Geometry: final body of the model. Coordinates: model frame, mm. Face numbers are marked on the shaded views. A direction names the side the tool comes from. Give positions to 0.01 mm unless a question says otherwise; leave off trailing zeros. Write each loop counter-clockwise with the first axis right and the second up, starting at its lowest first coordinate (ties: lowest second). Pieces come first, ordered by that corner, then holes.
Q1. Section B-B (y = 12.7). Return the cut outline in (x, z) (1 decimal).
Q2. Line query: line 1 (Y direction, x = 24.6, z = -5.92); line 2 (X direction, y = 0.75, z = 0) (3 decimals); line 3 (Y direction, x = 17.5, z = 7.25) (3 decimals). Output: solid intervals per line, ascending.
Q3. Reachability of the marked faces 1 and 2 from +Z, -Z, +X, -X, +Y, -Y: full face, straight path, thin tool, end or side. Return the list, or none.
Q4. Section C-C (x = 15). Return the cut outline in (y, z) (3 decimals), plus the area to 3 significant figures.
Q5. Section A-A (z = 0). State how many separate pieces and enclosed holes the cut face has, plus the area to 3 significant figures.
Q6. Pin query (flat end, axial travel): pin 1 Ø4 at (y, z) = (31.75, -5.92) entering from +X; pin 2 Ø4 at (x, z) = (15.58, 7.36) entering from +Y (3 decimals); pin 3 Ø2.5 at (x, z) = (15.58, -7.36) entering from -Y; pin 4 Ø12 at (y, z) = (15, 6.5) entering from -X (3 decimals). Return the tip coordinate at first contact, or that it passes through.
from build123d import *

# Parameters (mm, degrees)
BOSS_EXTRUDE1_DEPTH = 11
FILLET1_R           = 1.5875
SKETCH3_W           = 24.423912887
SKETCH3_H           = 26.552361768
CUT_EXTRUDE1_DEPTH  = 61.908127536
SKETCH4_R           = 1.5
SKETCH4_R_2         = 6.5
SKETCH4_W           = 25.825
SKETCH4_H           = 22
CUT_EXTRUDE2_DEPTH  = 53.363751775
SKETCH5_R           = 1.5875
CUT_EXTRUDE3_DEPTH  = 53.158921816


with BuildPart() as part:
    # Sketch2 → Boss-Extrude1 (new, symmetric)
    with BuildSketch(Plane.XY):
        Polygon((-25.4, 0), (25.4, 0), (25.4, 50.8), (22.225, 50.8), (22.225, 3.175), (-25.4, 3.175), align=None)
    extrude(amount=BOSS_EXTRUDE1_DEPTH, both=True)

    # Fillet1
    fillet1_edges = [part.edges().sort_by_distance(p)[0] for p in [
        (22.225, 3.175, 0),
    ]]
    fillet(fillet1_edges, radius=FILLET1_R)

    # Sketch3 → Cut-Extrude1 (cut, through all)
    with BuildSketch(Plane.XY.offset(11)):
        with Locations((18.271034128, 57.726180884)):
            Rectangle(SKETCH3_W, SKETCH3_H)
    extrude(amount=-CUT_EXTRUDE1_DEPTH, mode=Mode.SUBTRACT)

    # Sketch4 → Cut-Extrude2 (cut, through all)
    with BuildSketch(Plane.XZ):
        with Locations(Location((15.575, -7.361215932, 0), (0, 0, 270))):
            Circle(SKETCH4_R)
        with Locations(Location((11.325, 0, 0), (0, 0, 270))):
            Circle(SKETCH4_R_2)
        with Locations(Location((15.575, 7.361215932, 0), (0, 0, 270))):
            Circle(SKETCH4_R)
        with Locations((-12.4875, 0)):
            Rectangle(SKETCH4_W, SKETCH4_H)
        with Locations(Location((2.825, 0, 0), (0, 0, 270))):
            Circle(SKETCH4_R)
    extrude(amount=-CUT_EXTRUDE2_DEPTH, mode=Mode.SUBTRACT)

    # Sketch5 → Cut-Extrude3 (cut, through all)
    with BuildSketch(Plane(origin=(25.4, 0, 0), x_dir=(0, 0, -1), z_dir=(1, 0, 0))):
        with Locations((5.92, 31.75)):
            Circle(SKETCH5_R)
        with Locations((5.92, 12.7)):
            Circle(SKETCH5_R)
    extrude(amount=-CUT_EXTRUDE3_DEPTH, mode=Mode.SUBTRACT)


solid = part.part
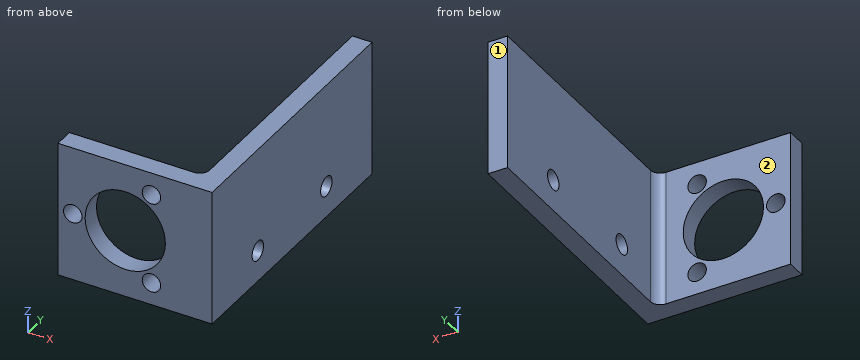
Computed:
1. outline: (22.2, -11) - (25.4, -11) - (25.4, -7.5) - (22.2, -7.5) - close; (22.2, -4.3) - (25.4, -4.3) - (25.4, 11) - (22.2, 11) - close
2. line 1: y = 0 to 11.11, 14.29 to 30.16, 33.34 to 44.45
2. line 2: x = 0.425 to 1.325, 4.325 to 4.825, 17.825 to 25.4
2. line 3: y = 0 to 3.175
3. face 1: +Z, -Z, +X, -X, +Y
3. face 2: +Z, -Z, -X, +Y
4. outline: (0, -11) - (3.175, -11) - (3.175, -8.747) - (0, -8.747) - close; (0, -5.976) - (3.175, -5.976) - (3.175, -5.361) - (0, -5.361) - close; (0, 5.361) - (3.175, 5.361) - (3.175, 5.976) - (0, 5.976) - close; (0, 8.747) - (3.175, 8.747) - (3.175, 11) - (0, 11) - close
4. area: 18.2 mm2
5. separate pieces: 3
5. enclosed holes: 0
5. area: 160 mm2
6. pin 1: stops at x = 25.4
6. pin 2: stops at y = 3.175
6. pin 3: passes through
6. pin 4: stops at x = 22.225
